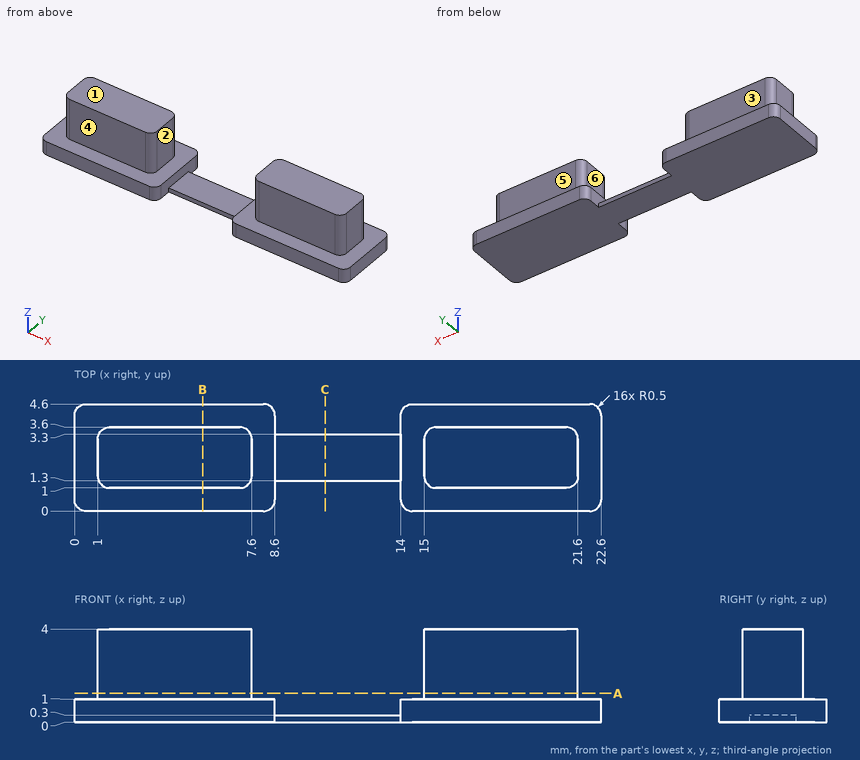
For this review, use the dimensioned drawing (mm, ordinates from the lowest corner) and the shaded views. A direction names the side the tool comes from. Coordinates: 2 decimals unless noted, no trailing zeros. Order: outer loops, then holes, each group sorted by start corner. A loop starts at its lowest first (then second) coordinate and runs counter-clockwise, first axis right, second up. Notation, with made-up numbers: (17.25, 26.25) - (22.25, 26.25) arc R24 ccw to (22.25, 61.25) - close; hole circle Ø11 at (-17, -26). An arc over 180 degrees is marked (long way). Answer as a JSON object with one key per item and string values. Group by question number.
1. We need section A-A on z = 1.25. State the section outline as (x, y) points.
2. For probe 1 along X at (y, z) = (3.95, 0.45); probe 2 along X at (y, z) = (1.6, 3); probe 3 along Z at (x, y) = (6.25, 4.45), list the stretches that pass through material, from the lowest coordinate up.
3. For the marked faces 1, 2, 3 and 4, list the 3-axis set-ups (+Z, -Z, +X, -X, +Y, -Y) from which the entire face can be reached by the end or side of a thin tool; tool diameter is ignored.
4. We need section C-C on x = 10.75. State the section outline as (y, z) points.
5. Clearance check with flat-ended pins moving along their axes: P1, Ø1.3, axis at y = 2.5, z = 2.5, coming from the -X side; P2, Ø0.5, axis at y = 2.5, z = 3, coming from the +X side; P3, Ø0.9, axis at x = 3.5, z = 2.5, coming from the +Y side. State where each tip first meets the part, or that it passes through.
6. The part is to be moulded in two halves that separate along X. For the marked faces 5 and 6, say which applies: pulls with the +X half, pulls with the -X half, needs draft (parallel to the pull), parting line crosses it, or undercut.
7. We need section B-B on x = 5.5. State the section outline as (y, z) points, then the cut area to 3 significant figures.
Final values:
{
 "1": {"outline": "(1, 1.5) arc R0.5 ccw to (1.5, 1) - (7.1, 1) arc R0.5 ccw to (7.6, 1.5) - (7.6, 3.1) arc R0.5 ccw to (7.1, 3.6) - (1.5, 3.6) arc R0.5 ccw to (1, 3.1) - close; (15, 1.5) arc R0.5 ccw to (15.5, 1) - (21.1, 1) arc R0.5 ccw to (21.6, 1.5) - (21.6, 3.1) arc R0.5 ccw to (21.1, 3.6) - (15.5, 3.6) arc R0.5 ccw to (15, 3.1) - close"},
 "2": {"probe 1": "0 to 8.6, 14 to 22.6", "probe 2": "1 to 7.6, 15 to 21.6", "probe 3": "0 to 1"},
 "3": {"face 1": "+Z, +X, -X, +Y, -Y", "face 2": "+Z, +Y, -Y", "face 3": "+Z, +X, -X, +Y", "face 4": "+Z, +X, -X, -Y"},
 "4": {"outline": "(1.3, 0) - (3.3, 0) - (3.3, 0.3) - (1.3, 0.3) - close"},
 "5": {"P1": "x = 1", "P2": "x = 21.6", "P3": "y = 3.6"},
 "6": {"face 5": "needs draft", "face 6": "undercut"},
 "7": {"outline": "(0, 0) - (4.6, 0) - (4.6, 1) - (3.6, 1) - (3.6, 4) - (1, 4) - (1, 1) - (0, 1) - close", "area": "12.4 mm²"}
}
